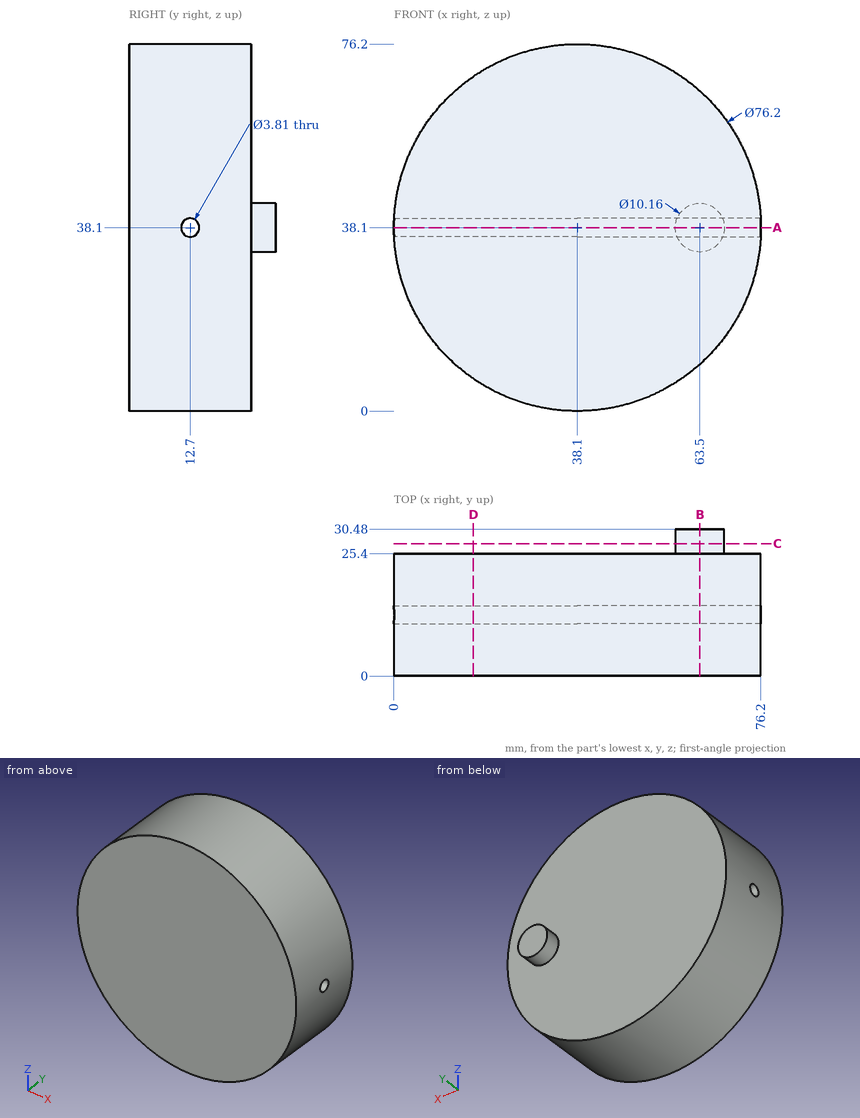
Geometry check sheet. Reference: drawing and pictorial views, mm from the part's lowest x, y, z. Give positions to 0.01 mm unless a question says otherwise; leave off trailing zeros. Order: outer loops, then holes, each group sorted by start corner. A loop starts at its lowest first (then second) coordinate and runs counter-clockwise, first axis right, second up. Notation, with made-up numbers: M 76,28.25 L 107,28.25 A24 cw 107,50.25 Z; hole C -33.75,52.5 d1. An arc over 180 degrees is marked long. Return JSON: item names as keys, results as strings. Group by question number.
1) Section check A-A on z = 38.1. Record the cut outline in (x, y) (3 decimals).
2) Go/stop test with flat-tipped pins: pin 1 Ø10 at (y, z) = (8.5, 23) entering from -X; pin 2 Ø3 at (x, z) = (54, 23.5) entering from +Y; pin 3 Ø2 at (x, y) = (10.5, 17.5) entering from +Z; pin 4 Ø3 at (y, z) = (12.7, 38.1) entering from +X. Record where each tip stops, or that it passes through.
3) Section check C-C on y = 27.5. Record the cut outline in (x, z), and give its area (3 significant figures).
4) Scan lines: line 1 (Y direction, x = 54, z = 38); line 2 (Y direction, x = 52.5, z = 21.5); line 3 (Z direction, x = 20, y = 12). Record each from-to range of solid material in increasing order.
5) Section check D-D on x = 16.5. Record the cut outline in (y, z) (1 decimal), and give its area (3 significant figures).
6) Section check B-B on x = 63.5. Record the cut outline in (y, z) (3 decimals).
Answer block:
{
 "1": {"outline": "M 0,0 L 76.2,0 L 76.2,10.795 L 0,10.795 Z; M 0,14.605 L 76.2,14.605 L 76.2,25.4 L 68.58,25.4 L 68.58,30.48 L 58.42,30.48 L 58.42,25.4 L 0,25.4 Z"},
 "2": {"pin 1": "stops at x = 1.36", "pin 2": "stops at y = 25.4", "pin 3": "stops at z = 65.38", "pin 4": "passes through"},
 "3": {"outline": "C 63.5,38.1 d10.16", "area": "81.1 mm^2"},
 "4": {"line 1": "y = 0 to 10.8, 14.6 to 25.4", "line 2": "y = 0 to 25.4", "line 3": "z = 4.57 to 36.33, 39.87 to 71.63"},
 "5": {"outline": "M 0,6.7 L 25.4,6.7 L 25.4,69.5 L 0,69.5 Z; hole C 12.7,38.1 d3.8", "area": "1,580 mm^2"},
 "6": {"outline": "M 0,9.702 L 25.4,9.702 L 25.4,33.02 L 30.48,33.02 L 30.48,43.18 L 25.4,43.18 L 25.4,66.498 L 0,66.498 Z; hole C 12.7,38.1 d3.81"}
}
